Autodesk Fusion 360 part; units mm, degrees
sketch "Sketch1" plane through (0, 0, 0) normal (0, 0, 1) x (1, 0, 0)
  circle A0 centre (0, 0) radius 31
  circle A1 centre (-18.5616, -18.5616) radius 1.75
  circle A2 centre (18.5616, 18.5616) radius 1.75
  circle A3 centre (-15, 0) radius 5
  line L0 (-18.5616, -18.5616) -> (-18.5616, -16.8116)
  circle A4 centre (15, 0) radius 5
  line L1 (0, 0) -> (0, 31)
  line L2 (0, 0) -> (31, 0)
  dimension "d1" = 62
  dimension "d6" = 3.5
  dimension "d10" = 15
  dimension "d11" = 10
extrude "Extrude1" add sketch "Sketch1" along normal blind 8 contours A0 A4 L1 L2 | A0 A4 L1 L2
ref_plane "WorkPlane1" through (0, 31, 0) normal (0, 1, 0) x (0, 0, 1)
sketch "Sketch2" plane through (0, 31, 0) normal (0, 1, 0) x (1, 0, 0)
  line L0 (0, 0) -> (0, -2.4162)
  circle A0 centre (0, -4.0162) radius 1.5
  dimension "d27" = 3
hole "Hole2" at (-15, 0, 8) direction (0, 0, -1) diameter 12 depth 18 tip angle 180
hole "Hole3" at (15, 0, 8) direction (0, 0, -1) diameter 12 depth 18 tip angle 180
hole "Hole4" at (0, 31, 4.0162) direction (0, -1, 0) diameter 3 depth 6 tip angle 180
pattern_circular "C-Pattern2" count 4 over 360 about axis through (0, 0, 1.75) along (0, 0, 1) of "Hole4"
extrude "Extrude2" add sketch "Sketch1" along normal blind 15 contours A1 | A2
Could you check a few things on this model? Use its own coordinates, in mm. A direction names the side the tool comes from. Round coordinates to 2 decimals unless told otherwise and drop trailing zeros. Order: outer loops, then holes, each group sorted by start corner. A loop starts at its lowest first (then second) coordinate and runs counter-clockwise, first axis right, second up.
(1) Imagine slicing it at A-A (y = 0). Write out the boundary of the cut face in (x, z).
Response values:
outline: (-31, 0) - (-21, 0) - (-21, 8) - (-31, 8) - (-31, 5.52) - (-25, 5.52) - (-25, 2.52) - (-31, 2.52) - close; (-9, 0) - (9, 0) - (9, 8) - (-9, 8) - close; (21, 0) - (31, 0) - (31, 2.52) - (25, 2.52) - (25, 5.52) - (31, 5.52) - (31, 8) - (21, 8) - close
(2) Please list where these lines run through material, in increasing order: line 1 along X through (y, z) = (0, 6.75); line 2 along X through (y, z) = (0, 5); line 3 along Z through (x, y) = (21.5, -16.5).
Response values:
line 1: x = -31 to -21, -9 to 9, 21 to 31
line 2: x = -25 to -21, -9 to 9, 21 to 25
line 3: z = 0 to 8
(3) Imagine slicing it at B-B (x = 11). Write out the boundary of the cut face in (y, z), plus the area to 3 significant figures.
Response values:
outline: (-28.98, 0) - (-4.47, 0) - (-4.47, 8) - (-28.98, 8) - close; (4.47, 0) - (28.98, 0) - (28.98, 8) - (4.47, 8) - close
area: 392 mm2
(4) Which directions (+Z, -Z, +X, -X, +Y, -Y) give clear straight access to the entire face, cutting with the end or side of a thin tool? Please do faces 5 (the flat face through (25, 0, 4)), 6 (the cylindrical face through (-27.958, 0.575, 5.402)), 7 (the flat face through (0, -25, 4)).
Response values:
face 5: +X
face 6: -X
face 7: -Y
(5) If we mould it in two halves opening along Z, with no side actions, what happens to faces 1 (the flat face through (0, 0, 8)), 2 (the cylindrical face through (9.05, 0.78, 3.94)), 3 (the flat face through (0, 0, 0)), 4 (the flat face through (-25, 0, 4))? For each: released by +Z, released by -Z, zero draft, split by the parting line, or undercut.
Response values:
face 1: released by +Z
face 2: zero draft
face 3: released by -Z
face 4: undercut
(6) Imagine slicing it at C-C (x = 0). Write out the boundary of the cut face in (y, z).
Response values:
outline: (-31, 0) - (31, 0) - (31, 2.52) - (25, 2.52) - (25, 5.52) - (31, 5.52) - (31, 8) - (-31, 8) - (-31, 5.52) - (-25, 5.52) - (-25, 2.52) - (-31, 2.52) - close
(7) I'm going to push flat-ended pins straight in: pin 1 (0.9 mm diameter, centred on x = 0, z = 4.5, fed in from +Y); pin 2 (12 mm diameter, centred on x = 18.5, y = -7, fed in from +Z); pin 3 (2.5 mm diameter, centred on x = -0.5, z = 4, fed in from -Y); pin 4 (11 mm diameter, centred on x = 15, y = 0, fed in from +Z). Where does each tip first touch, or does it pass through?
Response values:
pin 1: stops at y = 25
pin 2: stops at z = 8
pin 3: stops at y = -30.99
pin 4: passes through
(8) Imagine slicing it at D-D (z = 10.5). Write out the boundary of the cut face in (x, y), plus the area to 3 significant figures.
Response values:
outline: circle Ø3.5 at (-18.56, -18.56); circle Ø3.5 at (18.56, 18.56)
area: 19.2 mm2
